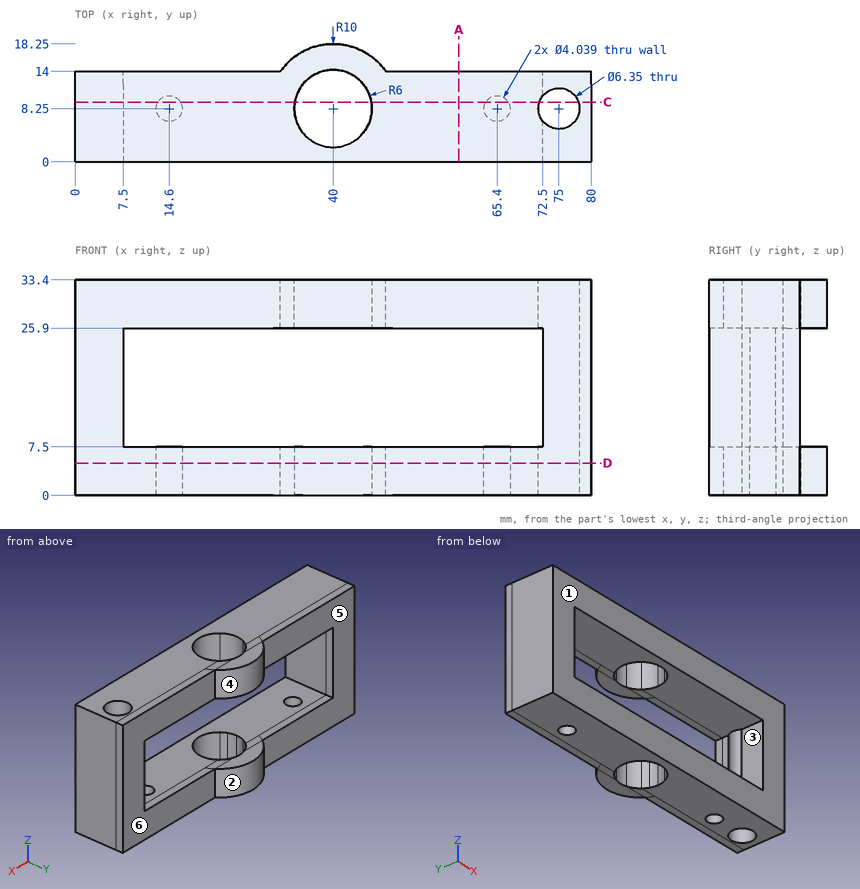
The drawing under review shows one solid part. Ordinate dimensions are in mm from its lowest x, y, z. A direction names the side the tool comes from. Round coordinates to 2 decimals unless told otherwise and drop trailing zeros. Loops run counter-clockwise (first coordinate to the right, second up) from the corner with the lowest first, then second, coordinate; pieces in that order, holes last. Notation, with made-up numbers: (-13.5, 44) - (-2.5, 44) arc R14 cw to (-2.5, 62) - close; hole circle Ø9 at (-4, 40.25). An arc over 180 degrees is marked (long way). One line per question, with ' | ' between items.
Q1. Take a section at D-D (z = 5). State how many separate pieces and enclosed holes the cut face has.
Taken from the geometry:
separate pieces: 1 | enclosed holes: 4
Q2. Tool access review of the marked faces 4, 5 and 6: name each direction out of +Z, -Z, +X, -X, +Y, -Y from which nothing blocks a thin tool from reaching the whole face with its end or side.
Taken from the geometry:
face 4: +Z, -Z, +Y | face 5: +Z, -Z, -X, +Y | face 6: +Z, -Z, +X, +Y
Q3. For line 1 along X through (y, z) = (8.5, 19.5) (1 decimal); line 2 along Z through (x, y) = (57, 10.75); line 3 along Y through (x, z) = (65.4, 1.75), list the stretches that pass through material, from the lowest coordinate up. Write a range as [from, to].
Taken from the geometry:
line 1: x = [0, 7.5], [78.2, 80] | line 2: z = [0, 7.5], [25.9, 33.4] | line 3: y = [0, 6.23], [10.27, 14]
Q4. Take a section at C-C (y = 9.25). Give the boundary of the cut face in (x, z) (1 decimal), and give its area (3 significant figures).
Taken from the geometry:
outline: (0, 0) - (12.8, 0) - (12.8, 7.5) - (7.5, 7.5) - (7.5, 25.9) - (34.1, 25.9) - (34.1, 33.4) - (0, 33.4) - close; (16.4, 0) - (34.1, 0) - (34.1, 7.5) - (16.4, 7.5) - close; (45.9, 0) - (63.6, 0) - (63.6, 7.5) - (45.9, 7.5) - close; (45.9, 25.9) - (72, 25.9) - (72, 33.4) - (45.9, 33.4) - close; (67.2, 0) - (72, 0) - (72, 7.5) - (67.2, 7.5) - close; (78, 0) - (80, 0) - (80, 33.4) - (78, 33.4) - close | area: 1,050 mm²
Q5. For pin 1 (2.5 mm diameter, centred on x = 14.6, y = 8.25, fed in from -Z), flat-tipped, find the tip position at first contact; note if it passes through.
Taken from the geometry:
pin 1: stops at z = 25.9
Q6. Take a section at A-A (x = 59.5). Give the boundary of the cut face in (y, z).
Taken from the geometry:
outline: (0, 0) - (14, 0) - (14, 7.5) - (0, 7.5) - close; (0, 25.9) - (14, 25.9) - (14, 33.4) - (0, 33.4) - close
Q7. The part is to be moulded in two halves that separate along X. For the marked faces 1, 2 and 3, say which applies: released by +X, released by -X, zero draft, split by the parting line, or undercut.
Taken from the geometry:
face 1: zero draft | face 2: split by the parting line | face 3: undercut
